from build123d import *

# Parameters (mm, degrees)
SKETCH1_W           = 138
SKETCH1_H           = 11.5
BOSS_EXTRUDE1_DEPTH = 17.8
SKETCH8_R           = 2
CUT_EXTRUDE4_DEPTH  = 11.5
SKETCH11_W          = 23
SKETCH11_H          = 11.5
CUT_EXTRUDE5_DEPTH  = 17.8
SKETCH14_W          = 80
SKETCH14_H          = 11.5
BOSS_EXTRUDE4_DEPTH = 10.5
CHAMFER1_SIZE       = 10.5
CHAMFER1_SIZE2      = 1.75
CHAMFER2_SIZE       = 10.5
CHAMFER2_SIZE2      = 1.75
SKETCH12_W          = 111
SKETCH12_H          = 7.5
CUT_EXTRUDE6_DEPTH  = 9.8
SKETCH13_W          = 55.5
SKETCH13_H          = 2
BOSS_EXTRUDE3_DEPTH = 7.5
FILLET1_R           = 7


with BuildPart() as part:
    # Sketch1 → Boss-Extrude1 (new body)
    with BuildSketch(Plane(origin=(0, 0, 0), x_dir=(1, 0, 0), z_dir=(0, 1, 0))):
        Rectangle(SKETCH1_W, SKETCH1_H)
    extrude(amount=-BOSS_EXTRUDE1_DEPTH)

    # Sketch8 → Cut-Extrude4 (cut)
    with BuildSketch(Plane.XY.offset(5.75)):
        with Locations((64.55, -13.35)):
            Circle(SKETCH8_R)
    extrude(amount=-CUT_EXTRUDE4_DEPTH, mode=Mode.SUBTRACT)

    # Sketch11 → Cut-Extrude5 (cut)
    with BuildSketch(Plane.XZ.offset(17.8)):
        with Locations((-57.5, 0)):
            Rectangle(SKETCH11_W, SKETCH11_H)
    extrude(amount=-CUT_EXTRUDE5_DEPTH, mode=Mode.SUBTRACT)

    # Sketch14 → Boss-Extrude4 (add)
    with BuildSketch(Plane(origin=(0, 0, 0), x_dir=(1, 0, 0), z_dir=(0, 1, 0))):
        with Locations((-6, 0)):
            Rectangle(SKETCH14_W, SKETCH14_H)
    extrude(amount=BOSS_EXTRUDE4_DEPTH)

    # Chamfer1
    chamfer1_edges = [part.edges().sort_by_distance(p)[0] for p in [
        (-6, 10.5, 5.75),
    ]]
    chamfer1_side = [part.faces().sort_by_distance(p)[0] for p in [
        (6.154026517, -4.745470138, 5.75),
    ]]
    chamfer(chamfer1_edges, length=CHAMFER1_SIZE, length2=CHAMFER1_SIZE2, reference=chamfer1_side[0])

    # Chamfer2
    chamfer2_edges = [part.edges().sort_by_distance(p)[0] for p in [
        (-6, 10.5, -5.75),
    ]]
    chamfer2_side = [part.faces().sort_by_distance(p)[0] for p in [
        (6.154026517, -4.745470138, -5.75),
    ]]
    chamfer(chamfer2_edges, length=CHAMFER2_SIZE, length2=CHAMFER2_SIZE2, reference=chamfer2_side[0])

    # Sketch12 → Cut-Extrude6 (cut)
    with BuildSketch(Plane.XZ.offset(17.8)):
        with Locations((11.5, 0)):
            Rectangle(SKETCH12_W, SKETCH12_H)
    extrude(amount=-CUT_EXTRUDE6_DEPTH, mode=Mode.SUBTRACT)

    # Sketch13 → Boss-Extrude3 (add)
    with BuildSketch(Plane.XY.offset(-3.75)):
        with Locations((-16.25, -13.3)):
            Rectangle(SKETCH13_W, SKETCH13_H)
    extrude(amount=BOSS_EXTRUDE3_DEPTH)

    # Fillet1
    # the kernel refuses this fillet: 7 mm, written as the material it takes off along each edge
    with BuildSketch(Plane(origin=(69, -17.8, 23.25), x_dir=(-1, 0, 0), z_dir=(0, 0, -1))) as fillet1_piece_1:
        with BuildLine():
            CenterArc((FILLET1_R, FILLET1_R), FILLET1_R, 180, 90)
            Line((0, FILLET1_R), (0, 0))
            Line((0, 0), (FILLET1_R, 0))
        make_face()
    extrude(amount=46.5, mode=Mode.SUBTRACT)


solid = part.part
Work out the finished part from the listing and answer in its coordinate system (mm). A direction names the side the tool comes from. Round coordinates to 2 decimals unless told otherwise and drop trailing zeros. Order: outer loops, then holes, each group sorted by start corner. A loop starts at its lowest first (then second) coordinate and runs counter-clockwise, first axis right, second up. Notation, with made-up numbers: M -40,-2 L -22,-2 A17 cw -22,14 Z; hole C 49.25,0.5 d10. An arc over 180 degrees is marked long. Put each result on its own line as item: value. Start each with the question number.
Q1. Section B-B, the plane x = 27 is taken. Write down the section's boundary in (y, z), and give its area (3 significant figures).
Q2. Flat-ended cylindrical pins translate along their axes: pin 1 (5 mm diameter, centred on y = 6, z = -2.5, fed in from +X); pin 2 (1.8 mm diameter, centred on y = -16, z = 0, fed in from +X); pin 3 (1.6 mm diameter, centred on y = -13.5, z = 1, fed in from +X); pin 4 (2.5 mm diameter, centred on x = 64.55, y = -13.35, fed in from -Z). Find the tip coordinate at first contact, or state that the pin passes through.
Q3. Section C-C, the plane z = -2.5 is taken. Write down the section's boundary in (x, y), and give its area (3 significant figures).
Q4. A tool of negligible diameter and unlimited length cuts with its end or side. For faces 1 (the flat face through (34, 5, 0)), 2 (the flat face through (-44, -16, 0)), 3 (the flat face through (-46, -4, 0)), 4 (the flat face through (11, -12, 3.75)), 5 (the cylindrical face through (67.78, -14.75, 0.08)), from which of +Z, -Z, +X, -X, +Y, -Y can it reach the whole face along a straight path? Write none if from no direction.
Q5. Section D-D, the plane x = 64.55 is taken. Write down the section's boundary in (y, z), and give its area (3 significant figures).
Q6. Straight lines are drawn through the part: L1, parallel to Z at x = -31.5, y = -16; L2, parallel to Y at x = -3.5, z = 2.5; L3, parallel to X at y = -11, z = 0. For each, find the intervals that lie inside material, in ascending order. Write a range as [from, to].
Q7. Section A-A, the plane x = -36 is taken. Write down the section's boundary in (y, z).
Q8. For a pull along Z with two mould halves and no side action, classify faces 6 (the flat face through (-6.56, 5.324, -4.863)), 7 (the flat face through (11, -8, 0)), 8 (the cylindrical face through (66.458, -12.749, -4.736)) as pulls with the +Z half, pulls with the -Z half, needs draft (parallel to the pull), parting line crosses it, or undercut.
Findings below:
1. outline: M -17.8,-5.75 L 0,-5.75 L 10.5,-4 L 10.5,4 L 0,5.75 L -17.8,5.75 L -17.8,3.75 L -8,3.75 L -8,-3.75 L -17.8,-3.75 Z
1. area: 234 mm^2
2. pin 1: stops at x = 34
2. pin 2: stops at x = 67.52
2. pin 3: stops at x = 68.74
2. pin 4: passes through
3. outline: M -46,-17.8 L -44,-17.8 L -44,-14.3 L 11.5,-14.3 L 11.5,-12.3 L -44,-12.3 L -44,-8 L 67,-8 L 67,-15.7 A7 ccw 69,-10.8 L 69,0 L 34,0 L 34,10.5 L -46,10.5 Z
3. area: 1,900 mm^2
4. face 1: +Z, -Z, +X, +Y
4. face 2: -Y
4. face 3: +Z, -Z, -X, +Y, -Y
4. face 4: none
4. face 5: +Z, -Z, +X, -Y
5. outline: M -17.32,-5.75 L -15.35,-5.75 L -15.35,-3.75 L -17.32,-3.75 Z; M -17.32,3.75 L -15.35,3.75 L -15.35,5.75 L -17.32,5.75 Z; M -11.35,-5.75 L 0,-5.75 L 0,5.75 L -11.35,5.75 L -11.35,3.75 L -8,3.75 L -8,-3.75 L -11.35,-3.75 Z
5. area: 113 mm^2
6. L1: z = [-5.75, -3.75], [3.75, 5.75]
6. L2: y = [-14.3, -12.3], [-8, 10.5]
6. L3: x = [-46, -44], [67, 69]
7. outline: M -17.8,-5.75 L 0,-5.75 L 10.5,-4 L 10.5,4 L 0,5.75 L -17.8,5.75 L -17.8,3.75 L -14.3,3.75 L -14.3,-3.75 L -17.8,-3.75 Z; hole M -12.3,-3.75 L -8,-3.75 L -8,3.75 L -12.3,3.75 Z
8. face 6: pulls with the -Z half
8. face 7: undercut
8. face 8: needs draft
